Geometry check sheet. Reference: the model listing, model coordinates, mm. A direction names the side the tool comes from. Round coordinates to 2 decimals unless told otherwise and drop trailing zeros. Write each loop counter-clockwise with the first axis right and the second up, starting at its lowest first coordinate (ties: lowest second). Pieces come first, ordered by that corner, then holes.
Item 1: Depth check by flat-ended pin: P1, Ø3, axis at x = -20.5, y = 2.5, coming from the -Z side. Enter the tip coordinate at first touch or a pass-through.
Item 2: Cross-section at C-C (x = -7). Enter the section's corners in (y, z).
Item 3: Cross-section at B-B (z = -3). Enter the section's corners in (x, y), then the cut area to 3 significant figures.
Item 4: Cross-section at A-A (z = 11.5). Enter the section's corners in (x, y), then the cut area to 3 significant figures.
Item 5: Scan lines: probe 1 along Y at (x, z) = (-3, 15); probe 2 along X at (y, z) = (-23.5, 12); probe 3 along Y at (x, z) = (-22.5, 15). Record each from-to range of solid material in increasing order.
Item 6: Draft check along Y on faces 4 (the face through (-4, -27.742, 15)), 5 (the face through (-27.288, -2, 16)), 6 (the face through (-19, 14, -7)). Enter one of: pulls with the +Y half, pulls with the -Y half, needs draft (parallel to the pull), parting line crosses it, or undercut.
Item 7: Cross-section at D-D (y = 9.5). Enter the section's corners in (x, z).
Item 8: Access from +Z, -Z, +X, -X, +Y, -Y to the whole of each face (thin tool, end or side, straight path). Record for faces 1 (the face through (-9, 4, 2)), 2 (the face through (-4, 24.258, 15)), 3 (the face through (-4, -1, 0)).
from build123d import *

# Parameters (mm, degrees)
F0_W     = 52
F0_H     = 52
F0_W_2   = 48
F0_H_2   = 48
F1_DEPTH = 30
F0_R     = 7.3390667627
F2_DEPTH = 7
F3_DEPTH = 2


with BuildPart() as f1:
    # F0 (on Top) → F1 (new body)
    with BuildSketch(Plane.XY):
        with Locations((-3.2878808908, -1.7417492345)):
            Rectangle(F0_W, F0_H)
        with Locations((-3.2878808908, -1.7417492345)):
            Rectangle(F0_W_2, F0_H_2, mode=Mode.SUBTRACT)
    extrude(amount=F1_DEPTH)



with BuildPart() as f1b:
    # F0 (on Top) → F1, piece 2 (new body)
    with BuildSketch(Plane.XY):
        with Locations((-3.2878808908, -1.7417492345)):
            Circle(F0_R)
    extrude(amount=F1_DEPTH)


with BuildPart() as f2:
    # F0 (on Top) → F2 (new body)
    with BuildSketch(Plane.XY):
        with BuildLine():
            ThreePointArc((18.7121191092, 14.2582507655), (12.7121191092, 20.2582507655), (6.7121191092, 14.2582507655))
            Line((6.7121191092, 14.2582507655), (12.7121191092, 14.2582507655))
            Line((12.7121191092, 14.2582507655), (12.7121191092, 8.2582507655))
            ThreePointArc((12.7121191092, 8.2582507655), (16.9547597963, 10.0156100784), (18.7121191092, 14.2582507655))
        make_face()
        with BuildLine():
            Line((12.7121191092, 14.2582507655), (6.7121191092, 14.2582507655))
            ThreePointArc((6.7121191092, 14.2582507655), (8.4694784221, 10.0156100784), (12.7121191092, 8.2582507655))
            Line((12.7121191092, 8.2582507655), (12.7121191092, 14.2582507655))
        make_face()
    extrude(amount=-F2_DEPTH)


with BuildPart() as f2b:
    # F0 (on Top) → F2, piece 2 (new body)
    with BuildSketch(Plane.XY):
        with BuildLine():
            Line((-19.2878808908, 14.2582507655), (-13.2878808908, 14.2582507655))
            ThreePointArc((-13.2878808908, 14.2582507655), (-23.5305215779, 18.5008914526), (-19.2878808908, 8.2582507655))
            Line((-19.2878808908, 8.2582507655), (-19.2878808908, 14.2582507655))
        make_face()
        with BuildLine():
            ThreePointArc((-19.2878808908, 8.2582507655), (-15.0452402037, 10.0156100784), (-13.2878808908, 14.2582507655))
            Line((-13.2878808908, 14.2582507655), (-19.2878808908, 14.2582507655))
            Line((-19.2878808908, 14.2582507655), (-19.2878808908, 8.2582507655))
        make_face()
    extrude(amount=-F2_DEPTH)


with BuildPart() as f2c:
    # F0 (on Top) → F2, piece 3 (new body)
    with BuildSketch(Plane.XY):
        with BuildLine():
            ThreePointArc((18.7121191092, -17.7417492345), (16.9547597963, -13.4991085474), (12.7121191092, -11.7417492345))
            Line((12.7121191092, -11.7417492345), (12.7121191092, -17.7417492345))
            Line((12.7121191092, -17.7417492345), (6.7121191092, -17.7417492345))
            ThreePointArc((6.7121191092, -17.7417492345), (12.7121191092, -23.7417492345), (18.7121191092, -17.7417492345))
        make_face()
        with BuildLine():
            Line((12.7121191092, -17.7417492345), (12.7121191092, -11.7417492345))
            ThreePointArc((12.7121191092, -11.7417492345), (8.4694784221, -13.4991085474), (6.7121191092, -17.7417492345))
            Line((6.7121191092, -17.7417492345), (12.7121191092, -17.7417492345))
        make_face()
    extrude(amount=-F2_DEPTH)


with BuildPart() as f2d:
    # F0 (on Top) → F2, piece 4 (new body)
    with BuildSketch(Plane.XY):
        with BuildLine():
            ThreePointArc((-13.2878808908, -17.7417492345), (-15.0452402037, -13.4991085474), (-19.2878808908, -11.7417492345))
            Line((-19.2878808908, -11.7417492345), (-19.2878808908, -17.7417492345))
            Line((-19.2878808908, -17.7417492345), (-13.2878808908, -17.7417492345))
        make_face()
        with BuildLine():
            Line((-19.2878808908, -17.7417492345), (-19.2878808908, -11.7417492345))
            ThreePointArc((-19.2878808908, -11.7417492345), (-23.5305215779, -21.9843899216), (-13.2878808908, -17.7417492345))
            Line((-13.2878808908, -17.7417492345), (-19.2878808908, -17.7417492345))
        make_face()
    extrude(amount=-F2_DEPTH)


with BuildPart() as f1_1:
    add(f1.part)

    add(f1b.part)  # F3 merges F1b

    add(f2.part)  # F3 merges F2

    add(f2b.part)  # F3 merges F2b

    add(f2c.part)  # F3 merges F2c

    add(f2d.part)  # F3 merges F2d
    # F0 (on Top) → F3 (join)
    with BuildSketch(Plane.XY):
        with Locations((-3.2878808908, -1.7417492345)):
            Rectangle(F0_W_2, F0_H_2)
        with BuildLine():
            ThreePointArc((-19.2878808908, 8.2582507655), (-23.5305215779, 18.5008914526), (-13.2878808908, 14.2582507655))
            Line((-13.2878808908, 14.2582507655), (6.7121191092, 14.2582507655))
            ThreePointArc((6.7121191092, 14.2582507655), (12.7121191092, 20.2582507655), (18.7121191092, 14.2582507655))
            ThreePointArc((18.7121191092, 14.2582507655), (16.9547597963, 10.0156100784), (12.7121191092, 8.2582507655))
            Line((12.7121191092, 8.2582507655), (12.7121191092, -11.7417492345))
            ThreePointArc((12.7121191092, -11.7417492345), (16.9547597963, -13.4991085474), (18.7121191092, -17.7417492345))
            ThreePointArc((18.7121191092, -17.7417492345), (12.7121191092, -23.7417492345), (6.7121191092, -17.7417492345))
            Line((6.7121191092, -17.7417492345), (-13.2878808908, -17.7417492345))
            ThreePointArc((-13.2878808908, -17.7417492345), (-23.5305215779, -21.9843899216), (-19.2878808908, -11.7417492345))
            Line((-19.2878808908, -11.7417492345), (-19.2878808908, 8.2582507655))
        make_face(mode=Mode.SUBTRACT)
        with BuildLine():
            ThreePointArc((-13.2878808908, -17.7417492345), (-15.0452402037, -13.4991085474), (-19.2878808908, -11.7417492345))
            Line((-19.2878808908, -11.7417492345), (-19.2878808908, -17.7417492345))
            Line((-19.2878808908, -17.7417492345), (-13.2878808908, -17.7417492345))
        make_face()
        with BuildLine():
            Line((-19.2878808908, -17.7417492345), (-19.2878808908, -11.7417492345))
            ThreePointArc((-19.2878808908, -11.7417492345), (-23.5305215779, -21.9843899216), (-13.2878808908, -17.7417492345))
            Line((-13.2878808908, -17.7417492345), (-19.2878808908, -17.7417492345))
        make_face()
        with BuildLine():
            Line((6.7121191092, 14.2582507655), (-13.2878808908, 14.2582507655))
            ThreePointArc((-13.2878808908, 14.2582507655), (-15.0452402037, 10.0156100784), (-19.2878808908, 8.2582507655))
            Line((-19.2878808908, 8.2582507655), (-19.2878808908, -11.7417492345))
            ThreePointArc((-19.2878808908, -11.7417492345), (-15.0452402037, -13.4991085474), (-13.2878808908, -17.7417492345))
            Line((-13.2878808908, -17.7417492345), (6.7121191092, -17.7417492345))
            ThreePointArc((6.7121191092, -17.7417492345), (8.4694784221, -13.4991085474), (12.7121191092, -11.7417492345))
            Line((12.7121191092, -11.7417492345), (12.7121191092, 8.2582507655))
            ThreePointArc((12.7121191092, 8.2582507655), (8.4694784221, 10.0156100784), (6.7121191092, 14.2582507655))
        make_face()
        with Locations((-3.2878808908, -1.7417492345)):
            Circle(F0_R, mode=Mode.SUBTRACT)
        with BuildLine():
            Line((-19.2878808908, 14.2582507655), (-13.2878808908, 14.2582507655))
            ThreePointArc((-13.2878808908, 14.2582507655), (-23.5305215779, 18.5008914526), (-19.2878808908, 8.2582507655))
            Line((-19.2878808908, 8.2582507655), (-19.2878808908, 14.2582507655))
        make_face()
        with BuildLine():
            ThreePointArc((-19.2878808908, 8.2582507655), (-15.0452402037, 10.0156100784), (-13.2878808908, 14.2582507655))
            Line((-13.2878808908, 14.2582507655), (-19.2878808908, 14.2582507655))
            Line((-19.2878808908, 14.2582507655), (-19.2878808908, 8.2582507655))
        make_face()
        with BuildLine():
            ThreePointArc((18.7121191092, 14.2582507655), (12.7121191092, 20.2582507655), (6.7121191092, 14.2582507655))
            Line((6.7121191092, 14.2582507655), (12.7121191092, 14.2582507655))
            Line((12.7121191092, 14.2582507655), (12.7121191092, 8.2582507655))
            ThreePointArc((12.7121191092, 8.2582507655), (16.9547597963, 10.0156100784), (18.7121191092, 14.2582507655))
        make_face()
        with BuildLine():
            Line((12.7121191092, 14.2582507655), (6.7121191092, 14.2582507655))
            ThreePointArc((6.7121191092, 14.2582507655), (8.4694784221, 10.0156100784), (12.7121191092, 8.2582507655))
            Line((12.7121191092, 8.2582507655), (12.7121191092, 14.2582507655))
        make_face()
        with BuildLine():
            Line((12.7121191092, -17.7417492345), (12.7121191092, -11.7417492345))
            ThreePointArc((12.7121191092, -11.7417492345), (8.4694784221, -13.4991085474), (6.7121191092, -17.7417492345))
            Line((6.7121191092, -17.7417492345), (12.7121191092, -17.7417492345))
        make_face()
        with BuildLine():
            ThreePointArc((18.7121191092, -17.7417492345), (16.9547597963, -13.4991085474), (12.7121191092, -11.7417492345))
            Line((12.7121191092, -11.7417492345), (12.7121191092, -17.7417492345))
            Line((12.7121191092, -17.7417492345), (6.7121191092, -17.7417492345))
            ThreePointArc((6.7121191092, -17.7417492345), (12.7121191092, -23.7417492345), (18.7121191092, -17.7417492345))
        make_face()
        with Locations((-3.2878808908, -1.7417492345)):
            Circle(F0_R)
    extrude(amount=F3_DEPTH)


solid = f1_1.part
Resolved:
1. P1: stops at z = 0
2. outline: (-27.74, 0) - (24.26, 0) - (24.26, 30) - (22.26, 30) - (22.26, 2) - (4.59, 2) - (4.59, 30) - (-8.07, 30) - (-8.07, 2) - (-25.74, 2) - (-25.74, 30) - (-27.74, 30) - close
3. outline: circle Ø12 at (-19.29, -17.74); circle Ø12 at (-19.29, 14.26); circle Ø12 at (12.71, -17.74); circle Ø12 at (12.71, 14.26)
3. area: 452 mm2
4. outline: (-29.29, -27.74) - (22.71, -27.74) - (22.71, 24.26) - (-29.29, 24.26) - close; circle Ø14.68 at (-3.29, -1.74); hole (-27.29, -25.74) - (20.71, -25.74) - (20.71, 22.26) - (-27.29, 22.26) - close
4. area: 569 mm2
5. probe 1: y = -27.74 to -25.74, -9.08 to 5.59, 22.26 to 24.26
5. probe 2: x = -29.29 to -27.29, 20.71 to 22.71
5. probe 3: y = -27.74 to -25.74, 22.26 to 24.26
6. face 4: pulls with the -Y half
6. face 5: undercut
6. face 6: needs draft
7. outline: (-29.29, 0) - (-22.94, 0) - (-22.94, -7) - (-15.63, -7) - (-15.63, 0) - (9.06, 0) - (9.06, -7) - (16.37, -7) - (16.37, 0) - (22.71, 0) - (22.71, 30) - (20.71, 30) - (20.71, 2) - (-27.29, 2) - (-27.29, 30) - (-29.29, 30) - close
8. face 1: +Z
8. face 2: +Z, -Z, +X, -X, +Y
8. face 3: -Z
